The drawing under review shows one solid part. Ordinate dimensions are in mm from its lowest x, y, z. A direction names the side the tool comes from. Coordinates: 2 decimals unless noted, no trailing zeros. Write each loop counter-clockwise with the first axis right and the second up, starting at its lowest first coordinate (ties: lowest second). Pieces come first, ordered by that corner, then holes.
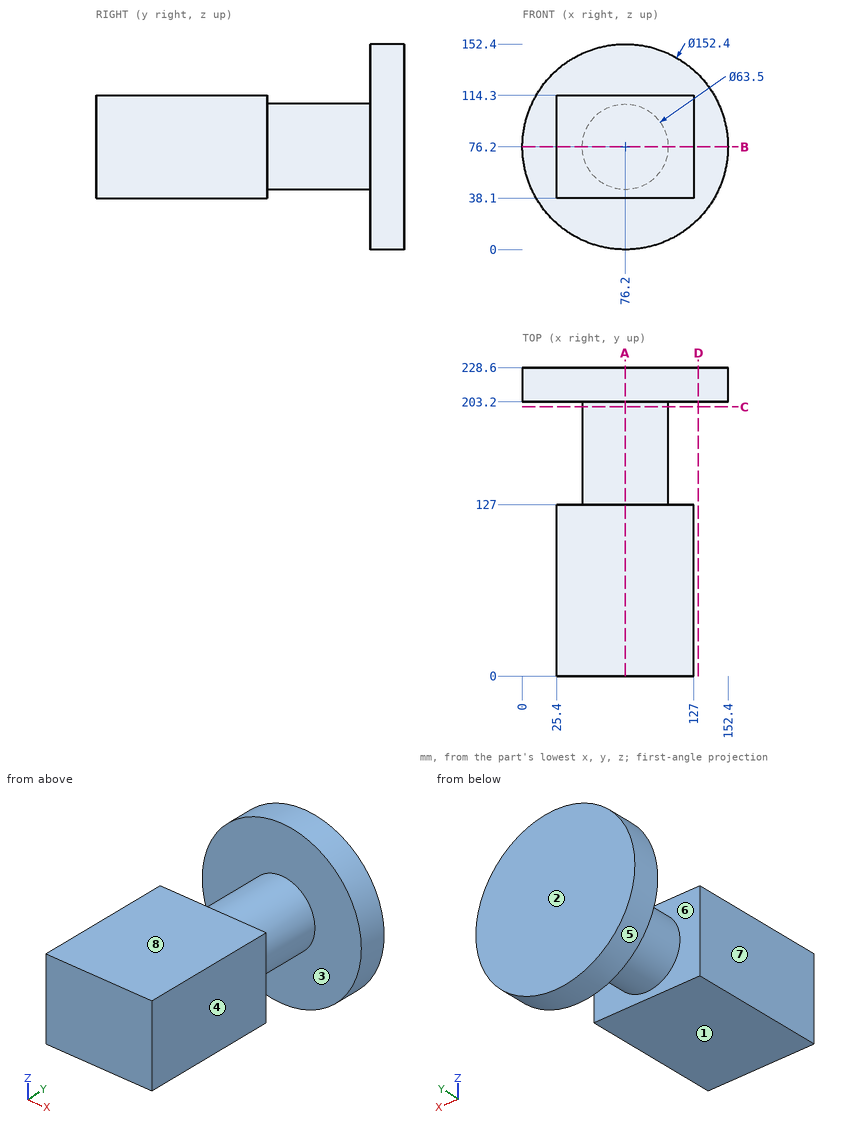
Q1. Add section D-D (x = 130.5). State the section outline as (y, z) points.
Ans:
outline: (203.2, 22.74) - (228.6, 22.74) - (228.6, 129.66) - (203.2, 129.66) - close
Q2. Add section A-A (x = 76.2). State the section outline as (y, z) points.
Ans:
outline: (0, 38.1) - (127, 38.1) - (127, 44.45) - (203.2, 44.45) - (203.2, 0) - (228.6, 0) - (228.6, 152.4) - (203.2, 152.4) - (203.2, 107.95) - (127, 107.95) - (127, 114.3) - (0, 114.3) - close
Q3. Clearance check with flat-ended pins moving along their axes: pin 1 Ø10 at (y, z) = (180, 73) entering from +X; pin 2 Ø10 at (x, y) = (43, 38.5) entering from -Z; pin 3 Ø1.5 at (x, y) = (113.5, 23.5) entering from +Z; pin 4 Ø8 at (y, z) = (155, 113.5) entering from -X. State where each tip first meets the part, or that it passes through.
Ans:
pin 1: stops at x = 107.95
pin 2: stops at z = 38.1
pin 3: stops at z = 114.3
pin 4: passes through
Q4. Draft analysis for pull direction Y (two halves, no side actions). For the marked faces 1, 2 and 3, state which applies: +Y half, -Y half, draft (parallel to the pull), parting line (faces both ways), or undercut.
Ans:
face 1: draft
face 2: +Y half
face 3: undercut
Q5. Tool access review of the marked faces 4, 5, 6, 7 and 8: name each direction out of +Z, -Z, +X, -X, +Y, -Y from which nothing blocks a thin tool from reaching the whole face with its end or side.
Ans:
face 4: +Z, -Z, +X, -Y
face 5: +Y, -Y
face 6: none
face 7: +Z, -Z, -X, -Y
face 8: +Z, +X, -X, -Y
Q6. For probe 1 along Y at (x, z) = (54, 47.5); probe 2 along Z at (x, y) = (37.5, 82); probe 3 along Y at (x, z) = (83.5, 137.5), list the stretches that pass through material, from the lowest coordinate up.
Ans:
probe 1: y = 0 to 127, 203.2 to 228.6
probe 2: z = 38.1 to 114.3
probe 3: y = 203.2 to 228.6
Q7. Add section B-B (z = 76.2). State the section outline as (x, y) points, then the cut area to 3 significant figures.
Ans:
outline: (0, 203.2) - (44.45, 203.2) - (44.45, 127) - (25.4, 127) - (25.4, 0) - (127, 0) - (127, 127) - (107.95, 127) - (107.95, 203.2) - (152.4, 203.2) - (152.4, 228.6) - (0, 228.6) - close
area: 21,600 mm2
Q8. Add section C-C (y = 199.5). State the section outline as (x, z) points.
Ans:
outline: circle Ø63.5 at (76.2, 76.2)
